Input: part model. Units: mm. Frame: model coordinates. A direction names the side the tool comes from. Coordinates: 2 decimals unless noted, no trailing zeros. Loops run counter-clockwise (first coordinate to the right, second up) from the corner with the lowest first, then second, coordinate; pieces in that order, holes last. Notation, with made-up numbers: (-8, 70) - (36, 70) arc R16 cw to (36, 74) - close; hole circle Ø5 at (62.5, 60.25). An arc over 180 degrees is marked (long way). Write item = value, one per line. Start each with the question number.
from build123d import *

# Parameters (mm, degrees)
EXTRUDE_1_DEPTH     = 2
SKETCH_3_R          = 2
EXTRUDE_2_DEPTH     = 3
SKETCH_4_R          = 1.5
CUT_EXTRUDE_1_DEPTH = 4
SKETCH_5_R          = 1
CUT_EXTRUDE_2_DEPTH = 4
SKETCH_6_R          = 0.5
CUT_EXTRUDE_3_DEPTH = 10


with BuildPart() as part:
    # 草图2 → 凸台-拉伸1 (new body)
    with BuildSketch(Plane.XY):
        with BuildLine():
            Line((-8.5, 2), (8.5, 2))
            ThreePointArc((8.5, 2), (10.5, 0), (8.5, -2))
            Line((8.5, -2), (-8.5, -2))
            ThreePointArc((-8.5, -2), (-10.5, 0), (-8.5, 2))
        make_face()
    extrude(amount=EXTRUDE_1_DEPTH)

    # 草图3 → 凸台-拉伸2 (add)
    with BuildSketch(Plane.XY.offset(2)):
        with Locations(Location((8.5, 0, 0), (0, 0, 90))):
            Circle(SKETCH_3_R)
    extrude(amount=EXTRUDE_2_DEPTH)

    # 草图4 → 切除-拉伸1 (cut)
    with BuildSketch(Plane.XY.offset(5)):
        with Locations((8.5, 0)):
            Circle(SKETCH_4_R)
    extrude(amount=-CUT_EXTRUDE_1_DEPTH, mode=Mode.SUBTRACT)

    # 草图5 → 切除-拉伸2 (cut)
    with BuildSketch(Plane.XY.offset(1)):
        with Locations((8.5, 0)):
            Circle(SKETCH_5_R)
    extrude(amount=-CUT_EXTRUDE_2_DEPTH, mode=Mode.SUBTRACT)

    # 草图6 → 切除-拉伸3 (cut)
    with BuildSketch(Plane(origin=(0, 0, 0), x_dir=(-1, 0, 0), z_dir=(0, 0, -1))):
        with Locations((-1.5, 0)):
            Circle(SKETCH_6_R)
        with Locations((1, 0)):
            Circle(SKETCH_6_R)
        with Locations((3.5, 0)):
            Circle(SKETCH_6_R)
        with Locations((6, 0)):
            Circle(SKETCH_6_R)
        with Locations((8.5, 0)):
            Circle(SKETCH_6_R)
    extrude(amount=-CUT_EXTRUDE_3_DEPTH, mode=Mode.SUBTRACT)


solid = part.part
Item 1: Cut plane C-C on y = 0.8. Return loops of the section in (x, z), plus the area to 3 significant figures.
Item 2: Cut plane B-B on x = 1.5. Return loops of the section in (y, z).
Item 3: Pull-direction query (X, two-part tool) for faces 1 (the cylindrical face through (2, 0, 1)), 2 (the flat face through (0, 2, 1)), 3 (the cylindrical face through (-9, 0, 1)), 4 (the cylindrical face through (10.452, -0.434, 3.021)); classes: pulls with the +X half, pulls with the -X half, needs draft (parallel to the pull), parting line crosses it, or undercut.
Item 4: Access query for faces 5 (the flat face through (0, -2, 1)), 6 (the cylindrical face through (7.3, -0.9, 3)). Directions: +Z, -Z, +X, -X, +Y, -Y. A direction counts if a zero-diameter tool reaches every point of the face in a straight line with its end or side. Return the directions, or none.
Item 5: Pin query (flat end, axial travel): pin 1 (2 mm diameter, centred on y = -1.5, z = 3, fed in from +X); pin 2 (2 mm diameter, centred on x = -4, y = -1, fed in from +Z); pin 3 (2 mm diameter, centred on y = 0, z = 3.5, fed in from -X). Return the tip coordinate at first contact, or that it passes through.
Item 6: Cut plane D-D on z = 2.2. Return loops of the section in (x, y).
Item 7: Cut plane A-A on y = 0. State how many separate pieces and enclosed holes the cut face has, plus the area to 3 significant figures.
Item 8: Ray query, line 1 (Y direction, x = 8.5, z = 3.8); line 2 (Y direction, x = -6, z = 1.85); line 3 (Z direction, x = 8.25, y = 1.4). Return the intervals inside material, ascending.
Recorded:
q1.outline = (-10.33, 0) - (7.9, 0) - (7.9, 1) - (7.23, 1) - (7.23, 5) - (6.67, 5) - (6.67, 2) - (-10.33, 2) - close; (9.1, 0) - (10.33, 0) - (10.33, 5) - (9.77, 5) - (9.77, 1) - (9.1, 1) - close
q1.area = 41.0 mm²
q2.outline = (-2, 0) - (-0.5, 0) - (-0.5, 2) - (-2, 2) - close; (0.5, 0) - (2, 0) - (2, 2) - (0.5, 2) - close
q3.face_1 = undercut
q3.face_2 = needs draft
q3.face_3 = undercut
q3.face_4 = parting line crosses it
q4.face_5 = +Z, -Z, +X, -X, -Y
q4.face_6 = +Z
q5.pin_1 = 10.44
q5.pin_2 = 2
q5.pin_3 = 6.5
q6.outline = circle Ø4 at (8.5, 0); hole circle Ø3 at (8.5, 0)
q7.separate_pieces = 7
q7.enclosed_holes = 0
q7.area = 30.0 mm²
q8.line_1 = -2 to -1.5, 1.5 to 2
q8.line_2 = -2 to -0.5, 0.5 to 2
q8.line_3 = 0 to 1
